```python
from build123d import *

# Parameters (mm, degrees)
EXTRUDE_1_DEPTH     = 3
CUT_EXTRUDE_4_DEPTH = 36.482389998
SKETCH_12_R         = 25
SKETCH_12_R_2       = 6.125
EXTRUDE_2_DEPTH     = 2.6
SKETCH_13_R         = 25
SKETCH_13_R_2       = 7.25
EXTRUDE_3_DEPTH     = 1.1
SKETCH_14_R         = 1.2
CUT_EXTRUDE_5_DEPTH = 36.984580031
FILLET_1_R          = 1


with BuildPart() as part:
    # 스케치1 → 보스-돌출1 (new body)
    with BuildSketch(Plane.XY):
        with BuildLine():
            Line((-5, -6.9), (-6.9, -6.9))
            Line((-6.9, -6.9), (-6.9, 6.9))
            Line((-6.9, 6.9), (6.9, 6.9))
            Line((6.9, 6.9), (6.9, -6.9))
            Line((6.9, -6.9), (5, -6.9))
            Line((5, -6.9), (5, -24.494897428))
            ThreePointArc((5, -24.494897428), (0, 25), (-5, -24.494897428))
            Line((-5, -24.494897428), (-5, -6.9))
        make_face()
    extrude(amount=EXTRUDE_1_DEPTH)

    # 스케치11 → 컷-돌출4 (cut, through all)
    with BuildSketch(Plane.XY.offset(3)):
        with BuildLine():
            Line((5.8, -1.8), (-5.8, -1.8))
            ThreePointArc((-5.8, -1.8), (-7.6, 0), (-5.8, 1.8))
            Line((-5.8, 1.8), (5.8, 1.8))
            ThreePointArc((5.8, 1.8), (7.6, 0), (5.8, -1.8))
        make_face()
    extrude(amount=-CUT_EXTRUDE_4_DEPTH, mode=Mode.SUBTRACT)

    # 스케치12 → 보스-돌출2 (add)
    with BuildSketch(Plane.XY.offset(3)):
        with Locations(Location((0, 0, 0), (0, 0, 258.463040967))):
            Circle(SKETCH_12_R)
        Circle(SKETCH_12_R_2, mode=Mode.SUBTRACT)
    extrude(amount=EXTRUDE_2_DEPTH)

    # 스케치13 → 보스-돌출3 (add)
    with BuildSketch(Plane.XY.offset(5.6)):
        with Locations(Location((0, 0, 0), (0, 0, 258.463040967))):
            Circle(SKETCH_13_R)
        Circle(SKETCH_13_R_2, mode=Mode.SUBTRACT)
    extrude(amount=EXTRUDE_3_DEPTH)

    # 스케치14 → 컷-돌출5 (cut, through all)
    with BuildSketch(Plane.XY.offset(6.7)):
        with Locations((19.485571585, -11.25)):
            Circle(SKETCH_14_R)
        with Locations((19.485571585, 11.25)):
            Circle(SKETCH_14_R)
        with Locations(Location((-19.485571585, 11.25, 0), (0, 0, 180))):
            Circle(SKETCH_14_R)
        with Locations(Location((-19.485571585, -11.25, 0), (0, 0, 180))):
            Circle(SKETCH_14_R)
    extrude(amount=-CUT_EXTRUDE_5_DEPTH, mode=Mode.SUBTRACT)

    # 필렛1
    fillet_1_edges = [part.edges().sort_by_distance(p)[0] for p in [
        (-5, -6.9, 1.5),
        (5, -6.9, 1.5),
    ]]
    fillet(fillet_1_edges, radius=FILLET_1_R)


solid = part.part
```
Model file for the job. Use its own axes, mm. A direction names the side the tool comes from. Give positions to 0.01 mm unless a question says otherwise; leave off trailing zeros. Loops run counter-clockwise (first coordinate to the right, second up) from the corner with the lowest first, then second, coordinate; pieces in that order, holes last. Notation, with made-up numbers: (87.5, -23.75) - (143.5, -23.75) arc R19 ccw to (143.5, -0.75) - close; hole circle Ø11 at (-24, 44). An arc over 180 degrees is marked (long way). One line per item, written item: value. Start each with the question number.
1. Probe L1, parallel to Y at x = 0, z = 6.1; L2, parallel to X at y = -4, z = 5; L3, parallel to X at y = -8, z = 2. List the from-to ranges inside material, lowest first. Write a range as from..to.
2. Which spindle directions (+Z, -Z, +X, -X, +Y, -Y) get a long thin tool onto all of the face, cutting with end or side? Do faces 1 (the flat face through (11, 1, 0)), 2 (the flat face through (-5, -16, 1)), 3 (the flat face through (6.9, 4, 1)), 4 (the cylindrical face through (-20.6, -10.8, 3.4)), 5 (the cylindrical face through (3.35, -6.43, 6.14)). Say none if no direction does.
3. Pin check, flat tips, straight feed: pin 1 (3.5 mm diameter, centred on y = 5, z = 2, fed in from +X); pin 2 (0.9 mm diameter, centred on x = -0.5, z = 1.5, fed in from -Y); pin 3 (5 mm diameter, centred on x = -3, y = 3, fed in from +Z); pin 4 (1.9 mm diameter, centred on x = 19.49, y = 11.25, fed in from -Z). Stop position of each tip, or through.
4. Slice it at B-B (y = -11.25). List the corners of the cut face in (x, z), plus the area to 3 significant figures.
5. Pull direction Y, two halves, no side cores. Call faces 6 (the cylindrical face through (-10.9, 22.5, 3.3)), 7 (the flat face through (5, -6, 6.7)), 8 (the cylindrical face through (3.293, 5.165, 4.282)): pulls with the +Y half, pulls with the -Y half, needs draft (parallel to the pull), parting line crosses it, or undercut.
6. Slice it at A-A (z = 2). List the corners of the cut face in (x, y), plus the area to 3 significant figures.
7. Slice it at C-C (x = -19). List the corners of the cut face in (y, z).
8. Slice it at D-D (y = 0). List the corners of the cut face in (x, z) (3 decimals), plus the area to 3 significant figures.
Solution:
1. L1: y = -25..-7.25, 7.25..25
1. L2: x = -24.68..-4.64, 4.64..24.68
1. L3: x = -23.69..-5, 5..23.69
2. face 1: -Z, +X, -X, +Y, -Y
2. face 2: -Z, -Y
2. face 3: -Z
2. face 4: +Z, -Z
2. face 5: +Z
3. pin 1: stops at x = 24.79
3. pin 2: stops at y = 6.9
3. pin 3: stops at z = 5.6
3. pin 4: passes through
4. outline: (-22.33, 0) - (-20.69, 0) - (-20.69, 6.7) - (-22.33, 6.7) - close; (-18.29, 0) - (-5, 0) - (-5, 3) - (5, 3) - (5, 0) - (18.29, 0) - (18.29, 6.7) - (-18.29, 6.7) - close; (20.69, 0) - (22.33, 0) - (22.33, 6.7) - (20.69, 6.7) - close
4. area: 237 mm^2
5. face 6: parting line crosses it
5. face 7: needs draft
5. face 8: undercut
6. outline: (-6.9, -6.9) - (-6.9, -1.42) arc R1.8 cw to (-6.9, 1.42) - (-6.9, 6.9) - (6.9, 6.9) - (6.9, 1.42) arc R1.8 cw to (6.9, -1.42) - (6.9, -6.9) - (6, -6.9) arc R1 ccw to (5, -7.9) - (5, -24.49) arc R25 ccw (long way) to (-5, -24.49) - (-5, -7.9) arc R1 ccw to (-6, -6.9) - close; hole circle Ø2.4 at (-19.49, -11.25); hole circle Ø2.4 at (-19.49, 11.25); hole circle Ø2.4 at (19.49, -11.25); hole circle Ø2.4 at (19.49, 11.25)
6. area: 1,570 mm^2
7. outline: (-16.25, 0) - (-12.35, 0) - (-12.35, 6.7) - (-16.25, 6.7) - close; (-10.15, 0) - (10.15, 0) - (10.15, 6.7) - (-10.15, 6.7) - close; (12.35, 0) - (16.25, 0) - (16.25, 6.7) - (12.35, 6.7) - close
8. outline: (-25, 0) - (-7.6, 0) - (-7.6, 3) - (-6.125, 3) - (-6.125, 5.6) - (-7.25, 5.6) - (-7.25, 6.7) - (-25, 6.7) - close; (6.125, 3) - (7.6, 3) - (7.6, 0) - (25, 0) - (25, 6.7) - (7.25, 6.7) - (7.25, 5.6) - (6.125, 5.6) - close
8. area: 242 mm^2
